from build123d import *

# Parameters (mm, degrees)
BASE_EXTRUDE_DEPTH = 11.1125
SKETCH2_R          = 3.2639
HOLE1_DEPTH        = 38.600633721
SKETCH3_R          = 3.2639
HOLE2_DEPTH        = 38.600633721


with BuildPart() as part:
    # Sketch1 → Base Extrude (new, symmetric)
    with BuildSketch(Plane(origin=(0, 0, 0), x_dir=(0, 0, -1), z_dir=(1, 0, 0))):
        with BuildLine():
            Line((-4.7625, 7.9375), (-4.7625, 20.6375))
            ThreePointArc((-4.7625, 20.6375), (-3.367596045, 24.005096045), (0, 25.4))
            Line((0, 25.4), (0, 0))
            Line((0, 0), (-25.4, 0))
            ThreePointArc((-25.4, 0), (-24.005096045, 3.367596045), (-20.6375, 4.7625))
            Line((-20.6375, 4.7625), (-7.9375, 4.7625))
            ThreePointArc((-7.9375, 4.7625), (-5.69243597, 5.69243597), (-4.7625, 7.9375))
        make_face()
    extrude(amount=BASE_EXTRUDE_DEPTH, both=True)

    # Sketch2 → Hole1 (cut, through all)
    with BuildSketch(Plane.XZ):
        with Locations(Location((0, 12.7, 0), (0, 0, 270))):
            Circle(SKETCH2_R)
    extrude(amount=-HOLE1_DEPTH, mode=Mode.SUBTRACT)

    # Sketch3 → Hole2 (cut, through all)
    with BuildSketch(Plane(origin=(0, 0, 0), x_dir=(-1, 0, 0), z_dir=(0, 0, -1))):
        with Locations(Location((0, 12.7, 0), (0, 0, 90))):
            Circle(SKETCH3_R)
    extrude(amount=-HOLE2_DEPTH, mode=Mode.SUBTRACT)


solid = part.part
Can you work these out from the model? Positions are in its coordinate system, mm. Coordinates: 2 decimals unless noted, no trailing zeros. Order: outer loops, then holes, each group sorted by start corner. A loop starts at its lowest first (then second) coordinate and runs counter-clockwise, first axis right, second up. Notation, with made-up numbers: M 52,-19 L 94,-19 A24 cw 94,1 Z; hole C 16,-31.75 d3. An arc over 180 degrees is marked long. Write item = value, one per line.
(1) If we mould it in two halves opening along Y, with no side actions, what happens to faces 1 (the face through (0.14, 9.44, 2.35)), 2 (the face through (0, 4.762, 17)), 3 (the face through (0, 17, 4.762))? For each: pulls with the +Y half, pulls with the -Y half, needs draft (parallel to the pull), parting line crosses it, or undercut.
Results are:
face_1 = undercut
face_2 = pulls with the +Y half
face_3 = needs draft
(2) For pin 1 Ø2 at (x, y) = (-7.5, 20) entering from +Z; pin 2 Ø10 at (x, z) = (-5.5, 16) entering from +Y, each with a flat end and sliding along its axis, tell me the tip position at first contact or that it passes through.
Results are:
pin_1 = 4.76
pin_2 = 4.76
(3) Suppose I cut it at B-B on x = 0. State how many separate pieces and enclosed holes the cut face has, plus the area to 3 significant figures.
Results are:
separate_pieces = 3
enclosed_holes = 0
area = 150 mm2
(4) I need wall thicknesses on line 1 along X through (y, z) = (12.7, 2.1); line 2 along Z through (x, y) = (4, 15). Which ranges of each line are inside material? Lowest first, please. Write a range as [from, to].
Results are:
line_1 = [-11.11, -3.26], [3.26, 11.11]
line_2 = [0, 4.76]
(5) Suppose I cut it at A-A on y = 12.7. Please give me the cut outline in (x, z).
Results are:
outline = M -11.11,0 L -3.26,0 L -3.26,4.76 L -11.11,4.76 Z; M 3.26,0 L 11.11,0 L 11.11,4.76 L 3.26,4.76 Z
